Source: CAD feature listing. Evaluate the final solid. Frame: model axes, mm. Face numbers are marked on the shaded views. A direction names the side the tool comes from. Give positions to 0.01 mm unless a question says otherwise; leave off trailing zeros. Loops run counter-clockwise (first coordinate to the right, second up) from the corner with the lowest first, then second, coordinate; pieces in that order, holes last. Notation, with made-up numbers: (-7.75, 74.25) -> (5.25, 74.25) arc R32 ccw to (5.25, 109.25) -> close; hole circle Ø4 at (-37, -14.5). An arc over 180 degrees is marked (long way). Return JSON: item names as keys, results as strings. Group by question number.
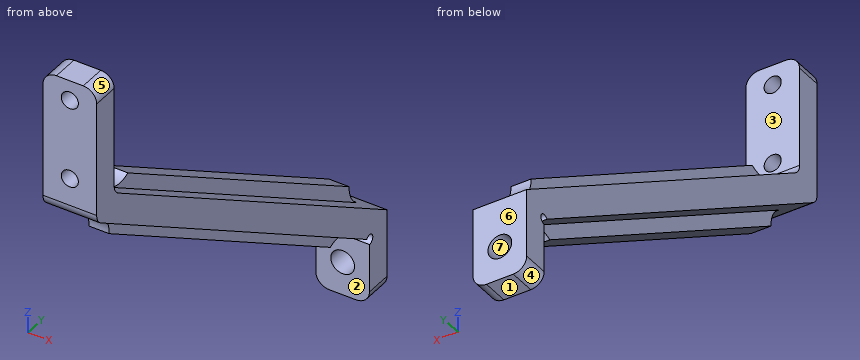
```python
from build123d import *

# Parameters (mm, degrees)
EXTRUDE_1_DEPTH          = 4
CUT_EXTRUDE_1_DEPTH      = 82.325026898
CUT_EXTRUDE_1_DEPTH_BACK = 82.325026898
SKETCH_2_R               = 1.275
CUT_EXTRUDE_2_DEPTH      = 85.433168838
CUT_EXTRUDE_2_DEPTH_BACK = 85.433168838
SKETCH_3_R               = 1.775
EXTRUDE_2_DEPTH          = 1.5
CUT_EXTRUDE_3_DEPTH      = 82.619605488
CUT_EXTRUDE_3_DEPTH_BACK = 82.619605488
SKETCH_5_R               = 0.75
FILLET_2_R               = 4
FILLET_3_R               = 2
FILLET_4_R               = 2


with BuildPart() as part:
    # 草图1 → 凸台-拉伸1 (new, symmetric)
    with BuildSketch(Plane(origin=(0, 0, 0), x_dir=(0, 0, -1), z_dir=(1, 0, 0))):
        Polygon((-18, 0), (0, 0), (39.807123819, 62.4), (52, 62.4), (52, 58.4), (42, 58.4), (2.192876181, -4), (-18, -4), align=None)
    extrude(amount=EXTRUDE_1_DEPTH, both=True)

    # 草图2 → 切除-拉伸1 (cut, two sides: drawn at the far end of the back side and taken through both)
    with BuildSketch(Plane(origin=(0, 0, 0), x_dir=(1, 0, 0), z_dir=(0, 1, 0)).offset(-CUT_EXTRUDE_1_DEPTH_BACK)):
        with Locations(Location((0, -3, 0), (0, 0, 270))):
            Circle(SKETCH_2_R)
        with Locations(Location((0, -15, 0), (0, 0, 270))):
            Circle(SKETCH_2_R)
    extrude(amount=CUT_EXTRUDE_1_DEPTH + CUT_EXTRUDE_1_DEPTH_BACK, mode=Mode.SUBTRACT)

    # 草图3 → 切除-拉伸2 (cut, two sides: drawn at the far end of the back side and taken through both)
    with BuildSketch(Plane(origin=(0, 62.4, 0), x_dir=(1, 0, 0), z_dir=(0, 1, 0)).offset(-CUT_EXTRUDE_2_DEPTH_BACK)):
        with Locations(Location((0, 47, 0), (0, 0, 270))):
            Circle(SKETCH_3_R)
    extrude(amount=CUT_EXTRUDE_2_DEPTH + CUT_EXTRUDE_2_DEPTH_BACK, mode=Mode.SUBTRACT)

    # 草图4 → 凸台-拉伸2 (add, symmetric)
    with BuildSketch(Plane(origin=(0, 0, 0), x_dir=(0, 0, -1), z_dir=(1, 0, 0))):
        Polygon((3.769025595, 5.908168553), (2.082903499, 6.983804308), (34.351976128, 57.567467201), (36.038098224, 56.491831447), align=None)
        Polygon((39.410342417, 54.340559938), (41.096464513, 53.264924184), (8.827391885, 2.681261291), (7.141269788, 3.756897045), align=None)
    extrude(amount=EXTRUDE_2_DEPTH, both=True)

    # 草图5 → 切除-拉伸3 (cut, two sides: drawn at the far end of the back side and taken through both)
    with BuildSketch(Plane(origin=(4, 0, 0), x_dir=(0, 0, -1), z_dir=(1, 0, 0)).offset(-CUT_EXTRUDE_3_DEPTH_BACK)):
        with Locations((42, 58.4)):
            Circle(SKETCH_5_R)
    extrude(amount=CUT_EXTRUDE_3_DEPTH + CUT_EXTRUDE_3_DEPTH_BACK, mode=Mode.SUBTRACT)

    # 圆角2
    # the kernel refuses this fillet: 4 mm, written as the material it adds along each edge
    with BuildSketch(Plane(origin=(-1.5, 3.756897045, -7.141269788), x_dir=(0, -0.8430610482191677, 0.5378178771439251), z_dir=(1, 0, 0)), Plane(origin=(-1.5, 56.491831447, -36.038098224), x_dir=(0, 0.8430610482191674, -0.5378178771439257), z_dir=(1, 0, 0))) as fillet_2_piece_1:
        with BuildLine():
            CenterArc((3.464101615, 4), FILLET_2_R, 210, 60)
            Line((0, 2), (-0.069282032, 1.96))
            ThreePointArc((-0.069282032, 1.96), (-0.08, 1), (-0.08, 0))
            Line((-0.08, 0), (0, -0.08))
            Line((0, -0.08), (3.464101615, -0.08))
            Line((3.464101615, -0.08), (3.464101615, 0))
        make_face()
    extrude(amount=3)
    with BuildSketch(Plane(origin=(-1.5, 5.908168553, -3.769025595), x_dir=(0, -0.8430610482191704, 0.5378178771439209), z_dir=(1, 0, 0)), Plane(origin=(-1.5, 54.340559938, -39.410342417), x_dir=(0, 0.8430610482191698, -0.5378178771439218), z_dir=(1, 0, 0))) as fillet_2_piece_2:
        with BuildLine():
            CenterArc((3.464101615, -4), FILLET_2_R, 90, 60)
            Line((0, -2), (-0.069282032, -1.96))
            ThreePointArc((-0.069282032, -1.96), (-0.08, -1), (-0.08, 0))
            Line((-0.08, 0), (0, 0.08))
            Line((0, 0.08), (3.464101615, 0.08))
            Line((3.464101615, 0.08), (3.464101615, 0))
        make_face()
    extrude(amount=3)

    # 圆角3
    fillet_3_edges = [part.edges().sort_by_distance(p)[0] for p in [
        (-4, -2, 18),
        (4, 60.4, -52),
        (4, -2, 18),
        (-4, 60.4, -52),
    ]]
    fillet(fillet_3_edges, radius=FILLET_3_R)

    # 圆角4
    fillet_4_edges = [part.edges().sort_by_distance(p)[0] for p in [
        (0, 0, 0),
        (0, -4, -2.192876181),
    ]]
    fillet(fillet_4_edges, radius=FILLET_4_R)


solid = part.part
```
1) Contact query for flat-ended pins moving along their axis: P1, Ø1.5, axis at x = -3, y = 3, coming from the -Z side; P2, Ø2.5, axis at x = -1, z = 8.5, coming from the +Y side; P3, Ø4, axis at x = 0, z = -47, coming from the +Y side; P4, Ø2, axis at x = 0, z = 15, coming from the -Y side. Output: stop coordinate, or through.
2) Cut plane C-C on y = 44. Return loops of the section in (x, z), then the cut area to 3 significant figures.
3) Cut plane A-A on z = -47. Return loops of the section in (x, y) (3 decimals), then the cut area to 3 significant figures.
4) Reachability of the marked faces 1, 2 and 3 from +Z, -Z, +X, -X, +Y, -Y: full face, straight path, thin tool, end or side. Return the list, or none.
5) Material intervals for line 1 (X direction, y = 59.8, z = -47) (3 decimals); line 2 (Y direction, x = -1, z = 6.5); line 3 (X direction, y = 42, z = -26), sorted ascending.
6) Cut plane D-D on z = -26. Return loops of the section in (x, y), then the cut area to 3 significant figures.
7) Mould query, pull axis X, two halves, no side actions, for the marked faces 4, 5, 6 and 7. Classes: released by +X, released by -X, zero draft, split by the parting line, or undercut.
8) Cut plane B-B on z = 15. Return loops of the section in (x, y) (3 decimals).
Calculated:
{
 "1": {"P1": "z = -7.14", "P2": "y = 0", "P3": "y = 62.4", "P4": "through"},
 "2": {"outline": "(-4, -32.81) -> (-1.5, -32.81) -> (-1.5, -35.19) -> (1.5, -35.19) -> (1.5, -32.81) -> (4, -32.81) -> (4, -28.07) -> (1.5, -28.07) -> (1.5, -25.7) -> (-1.5, -25.7) -> (-1.5, -28.07) -> (-4, -28.07) -> close", "area": "52.2 mm2"},
 "3": {"outline": "(-4, 58.4) -> (-1.775, 58.4) -> (-1.775, 62.4) -> (-4, 62.4) -> close; (1.775, 58.4) -> (4, 58.4) -> (4, 62.4) -> (1.775, 62.4) -> close", "area": "17.8 mm2"},
 "4": {"face 1": "-Z, +X, -X, +Y, -Y", "face 2": "-Z, +X, -X, -Y", "face 3": "+Z, +X, -X, +Y"},
 "5": {"line 1": "-4 to -1.775, 1.775 to 4", "line 2": "-4 to 0", "line 3": "-1.5 to 1.5"},
 "6": {"outline": "(-4, 33.32) -> (-1.5, 33.32) -> (-1.5, 29.6) -> (1.5, 29.6) -> (1.5, 33.32) -> (4, 33.32) -> (4, 40.76) -> (1.5, 40.76) -> (1.5, 44.48) -> (-1.5, 44.48) -> (-1.5, 40.76) -> (-4, 40.76) -> close", "area": "81.8 mm2"},
 "7": {"face 4": "released by -X", "face 5": "released by +X", "face 6": "zero draft", "face 7": "undercut"},
 "8": {"outline": "(-4, -4) -> (-1.275, -4) -> (-1.275, 0) -> (-4, 0) -> close; (1.275, -4) -> (4, -4) -> (4, 0) -> (1.275, 0) -> close"}
}
